Here's the drawing with two shaded views (mm, measured from the low corner). I have some questions. A direction names the side the tool comes from. Coordinates: 2 decimals unless noted, no trailing zeros. Loops run counter-clockwise (first coordinate to the right, second up) from the corner with the lowest first, then second, coordinate; pieces in that order, holes last.
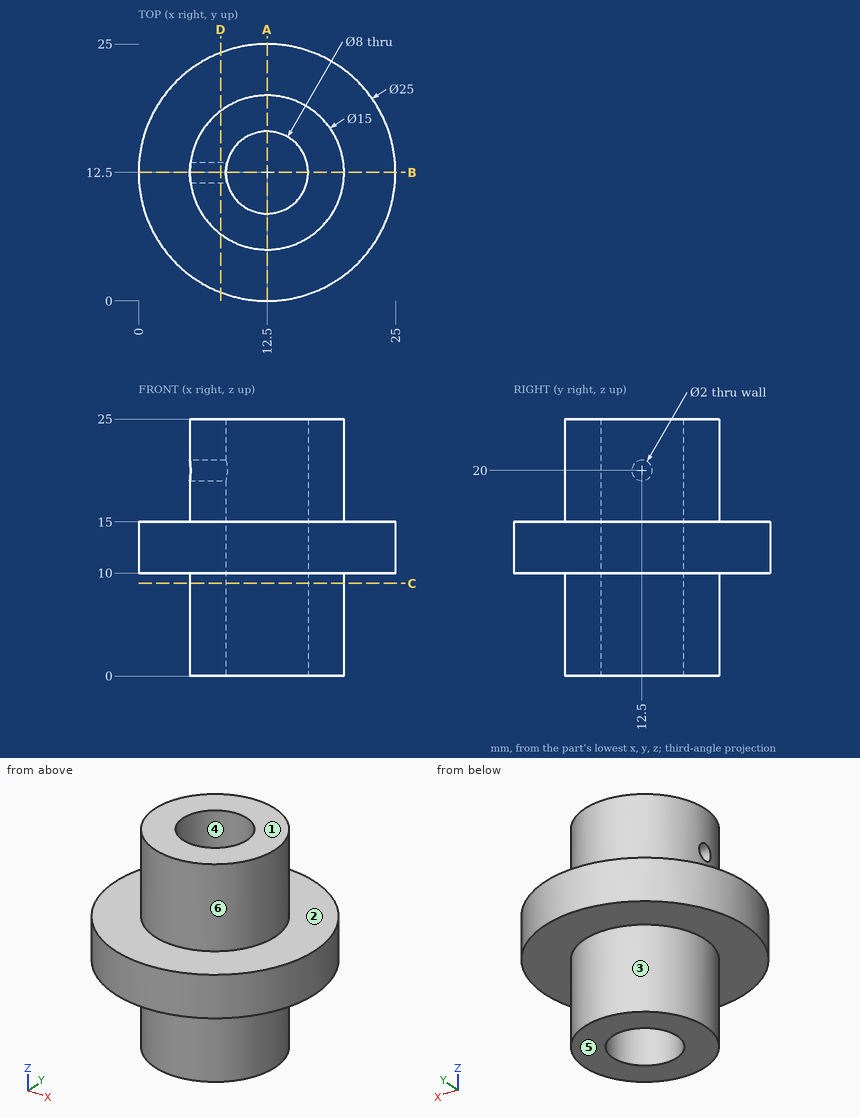
Q1. Please list where these lines run through material, in increasing order: probe 1 along Y at (x, z) = (12.5, 6.25); probe 2 along Z at (x, y) = (12.75, 3); probe 3 along Y at (x, z) = (7.1, 20).
Q2. For the marked faces 1, 2 and 3, which set-ups out of +Z, -Z, +X, -X, +Y, -Y let a thin tool reach every point of the face, with its end or its side?
Q3. Suppose I cut it at B-B on y = 12.5. Write out the boundary of the cut face in (x, z), and give its area (3 significant figures).
Q4. Suppose I cut it at D-D on x = 8. Write out the boundary of the cut face in (y, z).
Q5. Suppose I cut it at C-C on z = 9. Write out the boundary of the cut face in (x, y).
Q6. Will these pins go through, and if not, where does the flat tip stop? P1, Ø6, axis at y = 8, z = 10.5, coming from the -X side; P2, Ø3, axis at x = 4.5, y = 4.5, coming from the +Z side; P3, Ø3, axis at y = 4.5, z = 14.5, coming from the -X side.
Q7. Suppose I cut it at A-A on x = 12.5. Write out the boundary of the cut face in (y, z).
Q8. We'd pull the mould along X, two halves only. Please class the marked faces 4, 5 and 6: pulls with the +X half, pulls with the -X half, needs draft (parallel to the pull), parting line crosses it, or undercut.
Check values:
1. probe 1: y = 5 to 8.5, 16.5 to 20
1. probe 2: z = 10 to 15
1. probe 3: y = 7.3 to 11.5, 13.5 to 17.7
2. face 1: +Z, +X, -X, +Y, -Y
2. face 2: +Z
2. face 3: -Z
3. outline: (0, 10) - (5, 10) - (5, 0) - (8.5, 0) - (8.5, 19) - (5, 19) - (5, 15) - (0, 15) - close; (5, 21) - (8.5, 21) - (8.5, 25) - (5, 25) - close; (16.5, 0) - (20, 0) - (20, 10) - (25, 10) - (25, 15) - (20, 15) - (20, 25) - (16.5, 25) - close
3. area: 218 mm2
4. outline: (0.84, 10) - (6.5, 10) - (6.5, 0) - (18.5, 0) - (18.5, 10) - (24.16, 10) - (24.16, 15) - (18.5, 15) - (18.5, 25) - (6.5, 25) - (6.5, 15) - (0.84, 15) - close; hole circle Ø2 at (12.5, 20)
5. outline: circle Ø15 at (12.5, 12.5); hole circle Ø8 at (12.5, 12.5)
6. P1: stops at x = 0.09
6. P2: stops at z = 15
6. P3: stops at x = 1.82
7. outline: (0, 10) - (5, 10) - (5, 0) - (8.5, 0) - (8.5, 25) - (5, 25) - (5, 15) - (0, 15) - close; (16.5, 0) - (20, 0) - (20, 10) - (25, 10) - (25, 15) - (20, 15) - (20, 25) - (16.5, 25) - close
8. face 4: undercut
8. face 5: needs draft
8. face 6: parting line crosses it
